from build123d import *


with BuildPart() as part:
    # Sketch1 → Revolve1 (revolve)
    with BuildSketch(Plane.XY):
        with BuildLine():
            Line((6.35, -2.778125), (6.35, -8.334375))
            Line((6.35, -8.334375), (19.05, -8.334375))
            ThreePointArc((19.05, -8.334375), (15.554259867, 2.664147628), (6.35, 9.626137242))
            Line((6.35, 9.626137242), (6.35, 8.334375))
            Line((6.35, 8.334375), (6.35, 2.778125))
            Line((6.35, 2.778125), (3.302, 2.778125))
            Line((3.302, 2.778125), (3.302, 0))
            Line((3.302, 0), (3.302, -2.778125))
            Line((3.302, -2.778125), (6.35, -2.778125))
        make_face()
    revolve(axis=Axis((0, -2.778125, 0), (0, -1, 0)))


solid = part.part
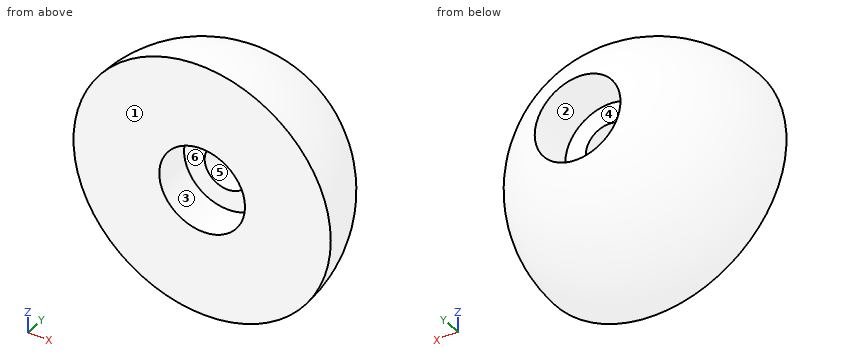
Could you check a few things on this model? Use its own coordinates, in mm. Face numbers are marked on the shaded views. A direction names the side the tool comes from. Coordinates: 2 decimals unless noted, no trailing zeros. Write each loop counter-clockwise with the first axis right and the second up, starting at its lowest first coordinate (ties: lowest second). Pieces come first, ordered by that corner, then holes. Notation, with made-up numbers: M 8.5,1 L 67.5,1 A25 cw 67.5,15 Z; hole C 51.5,75.25 d8. An arc over 180 degrees is marked long. One line per question, with ' | ' between items.
1) Imagine slicing it at A-A, the plane x = 0. Write out the boundary of the cut face in (y, z), and give its area (3 significant figures).
Checks:
outline: M -8.33,-19.05 A19.05 ccw 9.63,-6.35 L 2.78,-6.35 L 2.78,-3.3 L -2.78,-3.3 L -2.78,-6.35 L -8.33,-6.35 Z; M -8.33,6.35 L -2.78,6.35 L -2.78,3.3 L 2.78,3.3 L 2.78,6.35 L 9.63,6.35 A19.05 ccw -8.33,19.05 Z | area: 367 mm²
2) Imagine slicing it at C-C, the plane y = 0.5. Write out the boundary of the cut face in (x, z).
Checks:
outline: C 0,0 d33.76; hole C 0,0 d6.6
3) Imagine slicing it at D-D, the plane z = -4. Write out the boundary of the cut face in (x, y).
Checks:
outline: M -18.63,-8.33 L -4.93,-8.33 L -4.93,-2.78 L 4.93,-2.78 L 4.93,-8.33 L 18.63,-8.33 A18.63 ccw 4.93,9.63 L 4.93,2.78 L -4.93,2.78 L -4.93,9.63 A18.63 ccw Z
4) For pin 1 Ø7.5 at (x, z) = (0, 0) entering from +Y; pin 2 Ø2 at (x, y) = (3, -3) entering from -Z; pin 3 Ø3 at (y, z) = (0.5, 12.5) entering from -X; pin 4 Ø14 at (x, z) = (0, 0.5) entering from -Y, each with a flat end and sliding along its axis, tell me the tip position at first contact or that it passes through.
Checks:
pin 1: y = 2.78 | pin 2: z = -18.35 | pin 3: x = -13.13 | pin 4: y = -8.33
5) Imagine slicing it at B-B, the plane z = 0. Write out the boundary of the cut face in (x, y).
Checks:
outline: M -19.05,-8.33 L -6.35,-8.33 L -6.35,-2.78 L -3.3,-2.78 L -3.3,2.78 L -6.35,2.78 L -6.35,9.63 A19.05 ccw Z; M 3.3,-2.78 L 6.35,-2.78 L 6.35,-8.33 L 19.05,-8.33 A19.05 ccw 6.35,9.63 L 6.35,2.78 L 3.3,2.78 Z
6) If we mould it in two halves opening along Z, with no side actions, what happens to the marked faces 1, 2 and 3? For each: released by +Z, released by -Z, zero draft, split by the parting line, or undercut.
Checks:
face 1: zero draft | face 2: undercut | face 3: undercut
7) For the marked faces 4, 5 and 6, which set-ups out of +Z, -Z, +X, -X, +Y, -Y let a thin tool reach every point of the face, with its end or its side?
Checks:
face 4: +Y | face 5: +Y, -Y | face 6: -Y
8) I need wall thicknesses on probe 1 along Z at (x, y) = (-2.5, 0); probe 2 along Z at (x, y) = (0, -6.85); probe 3 along X at (y, z) = (0.25, -0.5). Which ranges of each line are inside material? Lowest first, please. Write a range as [from, to].
Checks:
probe 1: [-16.95, -2.16], [2.16, 16.95] | probe 2: [-18.99, -6.35], [6.35, 18.99] | probe 3: [-17, -3.26], [3.26, 17]
